from build123d import *

# Parameters (mm, degrees)
SKETCH_1_R          = 1.7
EXTRUDE_1_DEPTH     = 10
CUT_EXTRUDE_1_DEPTH = 37
SKETCH_3_W          = 3
SKETCH_3_H          = 5.795399196
SKETCH_3_W_2        = 5.804634465
SKETCH_3_H_2        = 3.015219691
SKETCH_3_H_3        = 5.79316294
CUT_EXTRUDE_2_DEPTH = 8
SKETCH_5_R          = 1.7
CUT_EXTRUDE_3_DEPTH = 35
CUT_EXTRUDE_START   = -35
SKETCH_6_R          = 1.7
CUT_EXTRUDE_4_DEPTH = 35
CUT_EXTRUDE_5_DEPTH = 10
SKETCH_9_R          = 5
CUT_EXTRUDE_6_DEPTH = 10
SKETCH_10_W         = 10
SKETCH_10_H         = 10.755893821
CUT_EXTRUDE_7_DEPTH = 7
SKETCH_13_W         = 10.237652643
SKETCH_13_H         = 10.849423333
CUT_EXTRUDE_8_DEPTH = 7


with BuildPart() as part:
    # Эскиз1 → Бобышка-Вытянуть1 (new body)
    with BuildSketch(Plane(origin=(0, 0, 0), x_dir=(0, 0, -1), z_dir=(1, 0, 0))):
        with BuildLine():
            Line((3, 0), (10.95312335, 0))
            ThreePointArc((10.95312335, 0), (12.757186433, 0.603052693), (13.835952782, 2.169762405))
            Line((13.835952782, 2.169762405), (21.800132861, 29.823741049))
            Line((21.800132861, 29.823741049), (21.800132861, 30.090305699))
            ThreePointArc((21.800132861, 30.090305699), (11.129115214, 41.472470419), (26.155254044, 37.272536706))
            Line((26.155254044, 37.272536706), (26.155045577, 20.433139704))
            ThreePointArc((26.155045577, 20.433139704), (29.083933995, 13.361991864), (36.155045576, 10.433015907))
            Line((36.155045576, 10.433015907), (83.844954424, 10.433015907))
            ThreePointArc((83.844954424, 10.433015907), (90.916066005, 13.361991864), (93.844954423, 20.433139704))
            Line((93.844954423, 20.433139704), (93.844745956, 37.272536706))
            ThreePointArc((93.844745956, 37.272536706), (108.870884786, 41.472470419), (98.199867139, 30.090305699))
            Line((98.199867139, 30.090305699), (98.199867139, 29.823741049))
            Line((98.199867139, 29.823741049), (106.164047218, 2.169762405))
            ThreePointArc((106.164047218, 2.169762405), (107.242813567, 0.603052693), (109.04687665, 0))
            Line((109.04687665, 0), (117, 0))
            ThreePointArc((117, 0), (119.121320344, 0.878679656), (120, 3))
            Line((120, 3), (120, 67))
            ThreePointArc((120, 67), (119.121320344, 69.121320344), (117, 70))
            Line((117, 70), (3, 70))
            ThreePointArc((3, 70), (0.878679656, 69.121320344), (0, 67))
            Line((0, 67), (0, 3))
            ThreePointArc((0, 3), (0.878679656, 0.878679656), (3, 0))
        make_face()
        with Locations((36, 65)):
            Circle(SKETCH_1_R, mode=Mode.SUBTRACT)
        with Locations((6, 65)):
            Circle(SKETCH_1_R, mode=Mode.SUBTRACT)
        with Locations((36, 31)):
            Circle(SKETCH_1_R, mode=Mode.SUBTRACT)
        with Locations((84, 31)):
            Circle(SKETCH_1_R, mode=Mode.SUBTRACT)
        with Locations((84, 65)):
            Circle(SKETCH_1_R, mode=Mode.SUBTRACT)
        with Locations((114, 65)):
            Circle(SKETCH_1_R, mode=Mode.SUBTRACT)
        with BuildLine():
            Line((47, 65), (73, 65))
            ThreePointArc((73, 65), (75.121320344, 64.121320344), (76, 62))
            Line((76, 62), (76, 41.380344056))
            ThreePointArc((76, 41.380344056), (75.121320344, 39.259023712), (73, 38.380344056))
            Line((73, 38.380344056), (47, 38.380344056))
            ThreePointArc((47, 38.380344056), (44.878679656, 39.259023712), (44, 41.380344056))
            Line((44, 41.380344056), (44, 62))
            ThreePointArc((44, 62), (44.878679656, 64.121320344), (47, 65))
        make_face(mode=Mode.SUBTRACT)
        with BuildLine():
            Line((48.512942473, 28.14808317), (71.745561711, 28.14808317))
            ThreePointArc((71.745561711, 28.14808317), (76.161679417, 23.731965464), (71.745561711, 19.315847758))
            Line((71.745561711, 19.315847758), (48.512942473, 19.315847758))
            ThreePointArc((48.512942473, 19.315847758), (44.096824767, 23.731965464), (48.512942473, 28.14808317))
        make_face(mode=Mode.SUBTRACT)
    extrude(amount=EXTRUDE_1_DEPTH)

    # Эскиз2 → Вырез-Вытянуть1 (cut)
    with BuildSketch(Plane(origin=(0, 70, 0), x_dir=(1, 0, 0), z_dir=(0, 1, 0))):
        with BuildLine():
            ThreePointArc((7, 60), (6.414213562, 61.414213562), (5, 62))
            Line((5, 62), (5, 60))
            Line((5, 60), (7, 60))
        make_face()
        with BuildLine():
            Line((5, 60), (5, 62))
            ThreePointArc((5, 62), (3.585786438, 58.585786438), (7, 60))
            Line((7, 60), (5, 60))
        make_face()
    extrude(amount=-CUT_EXTRUDE_1_DEPTH, mode=Mode.SUBTRACT)

    # Эскиз3 → Вырез-Вытянуть2 (cut)
    with BuildSketch(Plane.ZY):
        with Locations((-89.477143784, 21.994873796)):
            Rectangle(SKETCH_3_W, SKETCH_3_H)
        with Locations((-60.018321185, 34.987499707)):
            Rectangle(SKETCH_3_W_2, SKETCH_3_H_2)
        with Locations((-30.522856216, 21.995572621)):
            Rectangle(SKETCH_3_W, SKETCH_3_H_3)
    extrude(amount=-CUT_EXTRUDE_2_DEPTH, mode=Mode.SUBTRACT)

    # Эскиз5 → Вырез-Вытянуть3 (cut)
    with BuildSketch(Plane(origin=(0, 0, -120), x_dir=(-1, 0, 0), z_dir=(0, 0, -1))):
        with Locations(Location((-5, 22, 0), (0, 0, 292.826691269))):
            Circle(SKETCH_5_R)
    extrude(amount=-CUT_EXTRUDE_3_DEPTH, mode=Mode.SUBTRACT)

    # Эскиз6 → Вырез-Вытянуть4 (cut)
    with BuildSketch(Plane.XY.offset(CUT_EXTRUDE_START)):
        with Locations(Location((5, 22, 0), (0, 0, 247.173308731))):
            Circle(SKETCH_6_R)
    extrude(amount=CUT_EXTRUDE_4_DEPTH, mode=Mode.SUBTRACT)

    # Эскиз7 → Вырез-Вытянуть5 (cut)
    with BuildSketch(Plane.ZY):
        Polygon((-76.161679417, 23.731965464), (-83.844954424, 10.433015907), (-36.155045576, 10.433015907), (-44.096824767, 23.731965464), align=None)
    extrude(amount=-CUT_EXTRUDE_5_DEPTH, mode=Mode.SUBTRACT)

    # Эскиз9 → Вырез-Вытянуть6 (cut)
    with BuildSketch(Plane.ZY):
        with Locations((-99.973969782, 53.749400687)):
            Circle(SKETCH_9_R)
        with Locations((-20.026030218, 53.749400687)):
            Circle(SKETCH_9_R)
    extrude(amount=-CUT_EXTRUDE_6_DEPTH, mode=Mode.SUBTRACT)

    # Эскиз10 → Вырез-Вытянуть7 (cut)
    with BuildSketch(Plane.XY):
        with Locations((5, 22.092927416)):
            Rectangle(SKETCH_10_W, SKETCH_10_H)
    extrude(amount=-CUT_EXTRUDE_7_DEPTH, mode=Mode.SUBTRACT)

    # Эскиз13 → Вырез-Вытянуть8 (cut)
    with BuildSketch(Plane(origin=(0, 0, -120), x_dir=(-1, 0, 0), z_dir=(0, 0, -1))):
        with Locations((-5.118826322, 22.046162659)):
            Rectangle(SKETCH_13_W, SKETCH_13_H)
    extrude(amount=-CUT_EXTRUDE_8_DEPTH, mode=Mode.SUBTRACT)


solid = part.part
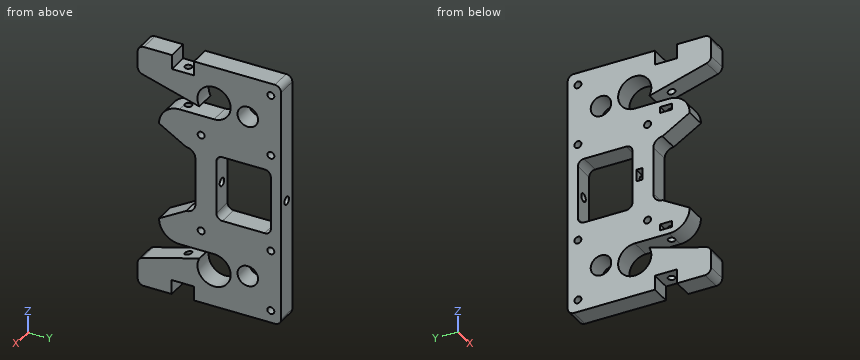
Geometry: final body of the model. Coordinates: model frame, mm. Give positions to 0.01 mm unless a question says otherwise; leave off trailing zeros. Loops run counter-clockwise (first coordinate to the right, second up) from the corner with the lowest first, then second, coordinate; pieces in that order, holes last. Notation, with made-up numbers: M -29,32.5 L 9,32.5 A24 cw 9,68.5 Z; hole C 43,29.25 d8. An arc over 180 degrees is marked long. Put each result on its own line as item: value.
1) Material intervals for L1, parallel to Y at x = 3.75, z = -6; L2, parallel to Z at x = 8.5, y = 25.5; L3, parallel to Z at x = 2.25, y = 46, sorted ascending. Write a range as from..to.
Computed values:
L1: y = 0..16.71, 27.47..63.3, 66.7..70
L2: z = -113..-99.45, -93.84..-75.79, -44.47..-26.16, -20.55..-7
L3: z = -120..-76, -44..0
2) First-contact query: P1, Ø2.5, axis at y = 22.5, z = -89.5, coming from the -X side; P2, Ø4, axis at y = 31, z = -36, coming from the -X side; P3, Ø3, axis at x = 5.5, y = 22.5, coming from the +Z side; P4, Ø2, axis at y = 65, z = -6, coming from the +X side. Flat tips, straight axial feed; report the tip coordinate or a pass-through.
Computed values:
P1: stops at x = 8
P2: stops at x = 0
P3: stops at z = -7
P4: passes through
3) Cut plane B-B, the plane y = 4.5. Return the cut outline in (x, z).
Computed values:
outline: M 0,-120 L 10,-120 L 10,-105.49 L 0,-105.49 Z; M 0,-14.51 L 10,-14.51 L 10,0 L 0,0 Z
4) Cut plane A-A, the plane z = -103. Return the cut outline in (x, y), plus the area to 3 significant figures.
Computed values:
outline: M 0,13.16 L 10,13.16 L 10,29.24 L 0,29.24 Z; M 0,45.3 L 10,45.3 L 10,49.77 L 0,49.77 Z; M 0,57.73 L 10,57.73 L 10,70 L 0,70 Z; hole C 5,22 d3.4
area: 319 mm^2
